```python
from build123d import *

# Parameters (mm, degrees)
IZIM1_R                     = 4
Y_KSEKLIK_EKSTR_ZYON1_DEPTH = 20
IZIM2_R                     = 6
Y_KSEKLIK_EKSTR_ZYON2_DEPTH = 28
IZIM3_R                     = 4
Y_KSEKLIK_EKSTR_ZYON3_DEPTH = 35
Y_KSEKLIK_EKSTR_ZYON4_START = -5
Y_KSEKLIK_EKSTR_ZYON4_DEPTH = 8
Y_KSEKLIK_EKSTR_ZYON5_START = -20
Y_KSEKLIK_EKSTR_ZYON5_DEPTH = 8


with BuildPart() as part:
    # Çizim1 → Yükseklik-Ekstrüzyon1 (new body)
    with BuildSketch(Plane(origin=(0, 0, 0), x_dir=(1, 0, 0), z_dir=(0, 1, 0))):
        with Locations(Location((0, 0, 0), (0, 0, 270))):
            Circle(IZIM1_R)
    extrude(amount=Y_KSEKLIK_EKSTR_ZYON1_DEPTH)

    # Çizim2 → Yükseklik-Ekstrüzyon2 (add)
    with BuildSketch(Plane(origin=(0, 20, 0), x_dir=(1, 0, 0), z_dir=(0, 1, 0))):
        with Locations(Location((0, 0, 0), (0, 0, 270))):
            Circle(IZIM2_R)
    extrude(amount=Y_KSEKLIK_EKSTR_ZYON2_DEPTH)

    # Çizim3 → Yükseklik-Ekstrüzyon3 (add)
    with BuildSketch(Plane(origin=(0, 48, 0), x_dir=(1, 0, 0), z_dir=(0, 1, 0))):
        with Locations(Location((0, 0, 0), (0, 0, 270))):
            Circle(IZIM3_R)
    extrude(amount=Y_KSEKLIK_EKSTR_ZYON3_DEPTH)

    # Çizim4 → Yükseklik-Ekstrüzyon4 (add)
    with BuildSketch(Plane.XZ.offset(Y_KSEKLIK_EKSTR_ZYON4_START)):
        Polygon((-6.308264839, 3.872314527), (-6.447035908, -3.631955985), (-0.017532542, -7.504270512), (6.550741893, -3.872314527), (6.689512962, 3.631955985), (0.260009596, 7.504270512), align=None)
    extrude(amount=-Y_KSEKLIK_EKSTR_ZYON4_DEPTH)

    # Çizim5 → Yükseklik-Ekstrüzyon5 (add)
    with BuildSketch(Plane(origin=(0, 83, 0), x_dir=(1, 0, 0), z_dir=(0, 1, 0)).offset(Y_KSEKLIK_EKSTR_ZYON5_START)):
        Polygon((6.773389455, -3.23334635), (6.186854806, 4.249254163), (-0.586534649, 7.482600513), (-6.773389455, 3.23334635), (-6.186854806, -4.249254163), (0.586534649, -7.482600513), align=None)
    extrude(amount=-Y_KSEKLIK_EKSTR_ZYON5_DEPTH)


solid = part.part
```
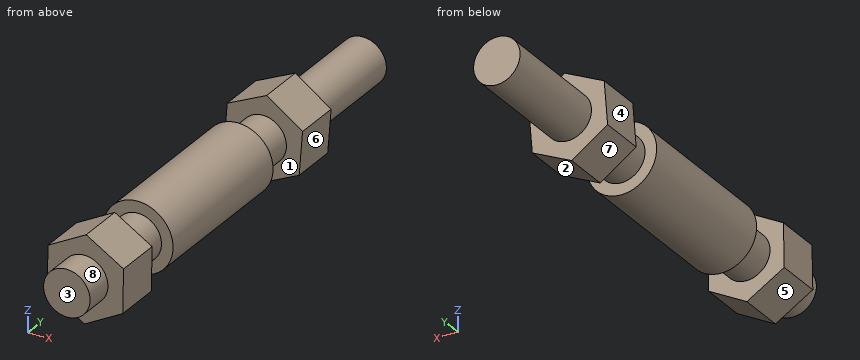
The listing builds one solid part. Answer for the finished solid, in the listing's coordinates (mm). Face numbers are marked on the shaded views. A direction names the side the tool comes from. Round coordinates to 2 decimals unless told otherwise and drop trailing zeros. Loops run counter-clockwise (first coordinate to the right, second up) from the corner with the lowest first, then second, coordinate; pieces in that order, holes last.
1) For a pull along Y with two mould halves and no side action, classify the marked faces 1, 2 and 3 as released by +Y, released by -Y, zero draft, split by the parting line, or undercut.
Outcome:
face 1: undercut
face 2: zero draft
face 3: released by -Y
2) A cutting plane is placed at B-B on z = 0. Determine the outline of the cut face in (x, y), plus the area to 3 significant figures.
Outcome:
outline: (-6.52, 55) - (-4, 55) - (-4, 48) - (-6, 48) - (-6, 20) - (-4, 20) - (-4, 13) - (-6.38, 13) - (-6.38, 5) - (-4, 5) - (-4, 0) - (4, 0) - (4, 5) - (6.62, 5) - (6.62, 13) - (4, 13) - (4, 20) - (6, 20) - (6, 48) - (4, 48) - (4, 55) - (6.52, 55) - (6.52, 63) - (4, 63) - (4, 83) - (-4, 83) - (-4, 63) - (-6.52, 63) - close
area: 856 mm2
3) A cutting plane is placed at C-C on x = 3.25. Determine the outline of the cut face in (y, z).
Outcome:
outline: (0, -2.33) - (5, -2.33) - (5, -5.7) - (13, -5.7) - (13, -2.33) - (20, -2.33) - (20, -5.04) - (48, -5.04) - (48, -2.33) - (55, -2.33) - (55, -5.65) - (63, -5.65) - (63, -2.33) - (83, -2.33) - (83, 2.33) - (63, 2.33) - (63, 5.65) - (55, 5.65) - (55, 2.33) - (48, 2.33) - (48, 5.04) - (20, 5.04) - (20, 2.33) - (13, 2.33) - (13, 5.7) - (5, 5.7) - (5, 2.33) - (0, 2.33) - close
4) For the marked faces 4, 5, 6, 7 and 8, determine the directions among +Z, -Z, +X, -X, +Y, -Y from which every point of the face is accessible in a straight line to the end or side of a thin tool.
Outcome:
face 4: +Z, -X, +Y
face 5: -Z, -X, -Y
face 6: -Z, +X, +Y
face 7: -Z, -X, +Y
face 8: -Y
5) A cutting plane is placed at A-A on x = -4.75. Determine the outline of the cut face in (y, z).
Outcome:
outline: (5, -4.65) - (13, -4.65) - (13, 4.73) - (5, 4.73) - close; (20, -3.67) - (48, -3.67) - (48, 3.67) - (20, 3.67) - close; (55, -4.62) - (63, -4.62) - (63, 4.94) - (55, 4.94) - close
6) Given P1, Ø1, axis at y = 65, z = -2.5, coming from the -X side; P2, Ø6, axis at y = 58, z = 1, coming from the -X side; P3, Ø1.5, axis at y = 17, z = -1.5, coming from the -X side, each flat-ended and moving along its own axis, determine where each tip first touches the part or whether it passes through.
Outcome:
P1: stops at x = -3.46
P2: stops at x = -6.68
P3: stops at x = -3.93
7) A cutting plane is placed at D-D on y = 14. Determine the outline of the cut face in (x, z).
Outcome:
outline: circle Ø8 at (0, 0)
8) Consider line 1 (Y direction, x = -2.25, z = 4); line 2 (Y direction, x = -1, z = -6); line 3 (X direction, y = 68.5, z = -1). Determine where each line is inside the solid, lowest interval first.
Outcome:
line 1: y = 5 to 13, 20 to 48, 55 to 63
line 2: y = 5 to 13, 55 to 63
line 3: x = -3.87 to 3.87
